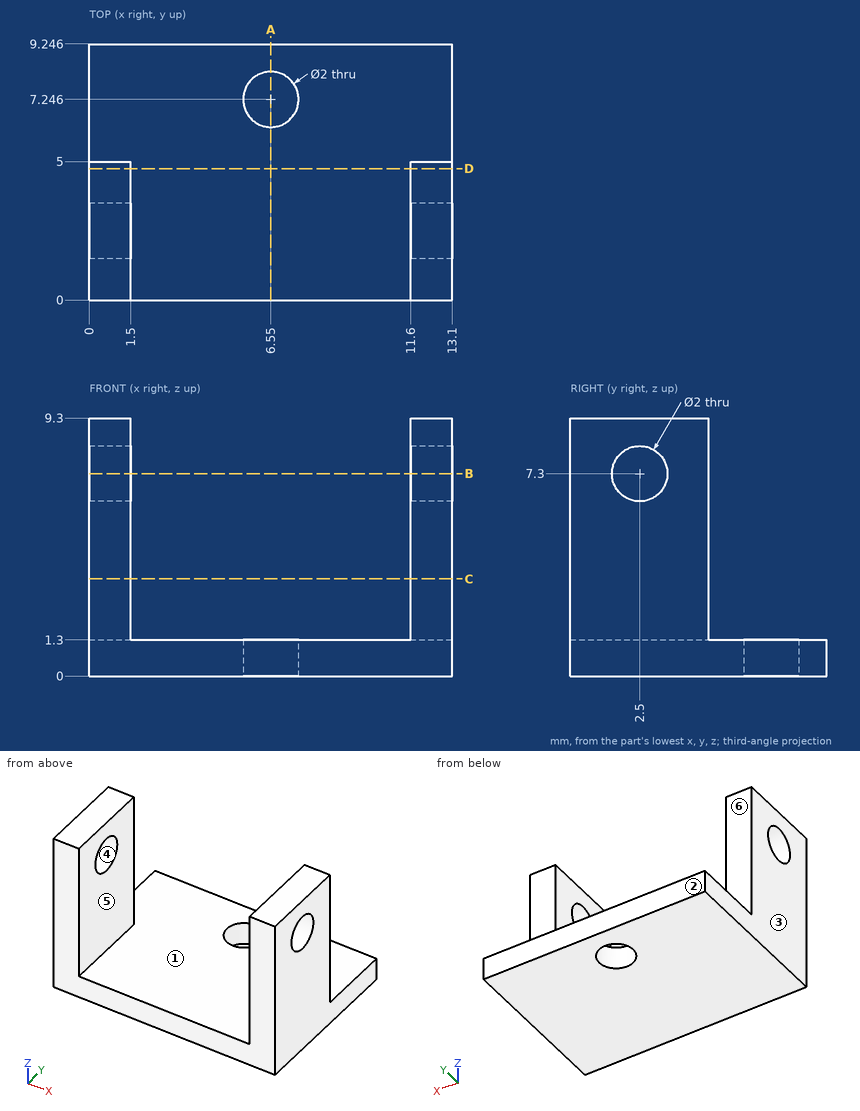
Part print with two shaded views. Sizes in mm from the minimum x, y, z corner. A direction names the side the tool comes from. Give positions to 0.01 mm unless a question says otherwise; leave off trailing zeros. Loops run counter-clockwise (first coordinate to the right, second up) from the corner with the lowest first, then second, coordinate; pieces in that order, holes last. Notation, with made-up numbers: (-31, 55) -> (20, 55) arc R19 ccw to (20, 63) -> close; hole circle Ø4 at (1.5, -2.75). An arc over 180 degrees is marked (long way). One line per question, with ' | ' between items.
Q1. Cut at D-D, the plane y = 4.75. Write the cut outline in (x, z).
Filled sheet:
outline: (0, 0) -> (13.1, 0) -> (13.1, 9.3) -> (11.6, 9.3) -> (11.6, 1.3) -> (1.5, 1.3) -> (1.5, 9.3) -> (0, 9.3) -> close
Q2. Pull direction X, two halves, no side cores. Call the marked faces 1, 2 and 3: pulls with the +X half, pulls with the -X half, needs draft (parallel to the pull), parting line crosses it, or undercut.
Filled sheet:
face 1: undercut | face 2: needs draft | face 3: pulls with the -X half
Q3. Cut at B-B, the plane z = 7.3. Write the cut outline in (x, y).
Filled sheet:
outline: (0, 0) -> (1.5, 0) -> (1.5, 1.5) -> (0, 1.5) -> close; (0, 3.5) -> (1.5, 3.5) -> (1.5, 5) -> (0, 5) -> close; (11.6, 0) -> (13.1, 0) -> (13.1, 1.5) -> (11.6, 1.5) -> close; (11.6, 3.5) -> (13.1, 3.5) -> (13.1, 5) -> (11.6, 5) -> close
Q4. Cut at A-A, the plane x = 6.55. Write the cut outline in (y, z) (1 decimal).
Filled sheet:
outline: (0, 0) -> (6.2, 0) -> (6.2, 1.3) -> (0, 1.3) -> close; (8.2, 0) -> (9.2, 0) -> (9.2, 1.3) -> (8.2, 1.3) -> close
Q5. Tool access for the marked faces 4, 5 and 6: list every direction of +Z, -Z, +X, -X, +Y, -Y with a clear straight run to the whole face (end or side of a thin tool).
Filled sheet:
face 4: +X, -X | face 5: +Z, +Y, -Y | face 6: +Z, +X, -X, +Y
Q6. Drop a flat-ended pin along its axis: pin 1 (1.6 mm diameter, centred on x = 12.5, z = 4.5, fed in from +Y). Give the stop position or say it passes through.
Filled sheet:
pin 1: stops at y = 5
Q7. Drill centre lines: line 1 along Y through (x, z) = (12.35, 7.3); line 2 along X through (y, z) = (4.5, 4); line 3 along Z through (x, y) = (11.25, 6). Where is each one in solid material? Low to high. Write a range as [from, to].
Filled sheet:
line 1: y = [0, 1.5], [3.5, 5] | line 2: x = [0, 1.5], [11.6, 13.1] | line 3: z = [0, 1.3]
Q8. Cut at C-C, the plane z = 3.5. Write the cut outline in (x, y).
Filled sheet:
outline: (0, 0) -> (1.5, 0) -> (1.5, 5) -> (0, 5) -> close; (11.6, 0) -> (13.1, 0) -> (13.1, 5) -> (11.6, 5) -> close
